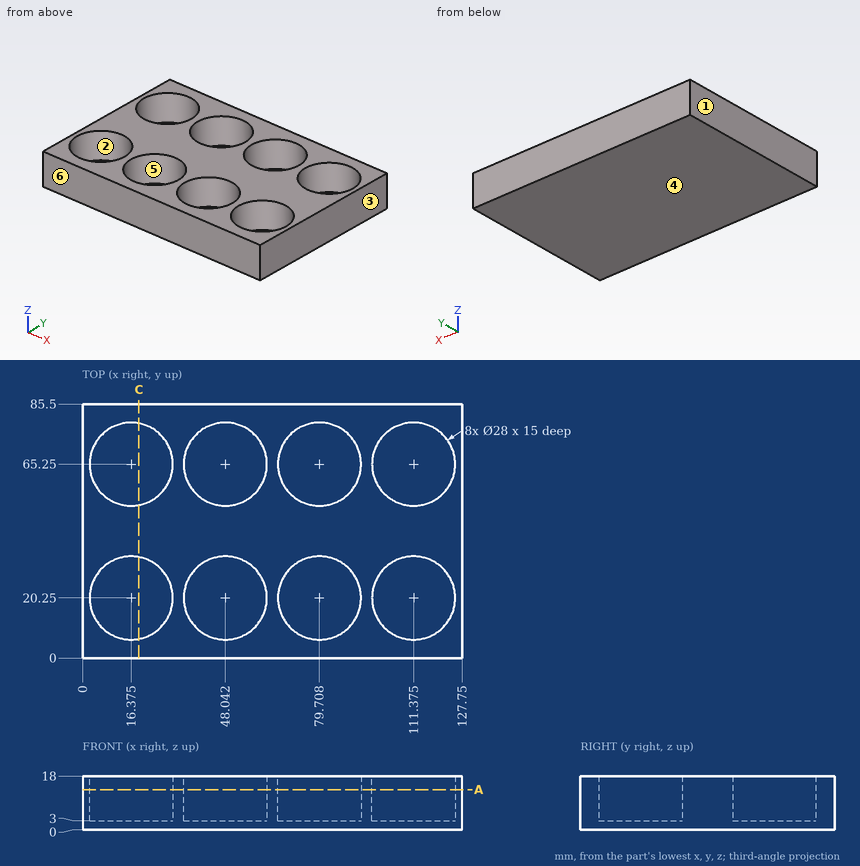
The figure shows three views and two pictorial views of one solid part (mm, origin at its lowest corner). Answer the questions. A direction names the side the tool comes from. Round coordinates to 2 decimals unless told otherwise and drop trailing zeros. Write each loop counter-clockwise with the first axis right and the second up, starting at its lowest first coordinate (ties: lowest second). Pieces come first, ordered by that corner, then holes. Notation, with made-up numbers: (-0.5, 4) - (6.5, 4) arc R27 cw to (6.5, 23) - close; hole circle Ø6 at (72.25, 57.25). An arc over 180 degrees is marked (long way). One line per question, with ' | ' between items. Start each with the question number.
1. Section A-A (z = 13.5) is taken. Give the number of separate pieces and of enclosed holes in the cut face, and give its area (3 significant figures).
2. For a pull along X with two mould halves and no side action, classify the marked faces 1, 2, 3 and 4 as +X half, -X half, draft (parallel to the pull), parting line (faces both ways), or undercut.
3. Find the intervals of material crossed by probe 1 along Y at (x, z) = (48.5, 16); probe 2 along Y at (x, z) = (118, 15.25); probe 3 along Z at (x, y) = (68, 17.5), in increasing order. Write a range as [from, to].
4. For the marked faces 5 and 6, determine the directions among +Z, -Z, +X, -X, +Y, -Y from which every point of the face is accessible in a straight line to the end or side of a thin tool.
5. Section C-C (x = 19) is taken. Determine the outline of the cut face in (y, z), and give its area (3 significant figures).
6. Each of these flat-tipped pins is pushed along its axis until it touches: pin 1 (14 mm diameter, centred on x = 75.5, y = 69, fed in from +Z); pin 2 (17 mm diameter, centred on x = 48.04, y = 20.25, fed in from -Z). Where does it stop, or does it pass through?
Filled in:
1) separate pieces: 1 | enclosed holes: 8 | area: 6,000 mm²
2) face 1: -X half | face 2: undercut | face 3: +X half | face 4: draft
3) probe 1: [0, 6.26], [34.24, 51.26], [79.24, 85.5] | probe 2: [0, 7.92], [32.58, 52.92], [77.58, 85.5] | probe 3: [0, 3]
4) face 5: +Z | face 6: +Z, -Z, +X, -X, -Y
5) outline: (0, 0) - (85.5, 0) - (85.5, 18) - (79, 18) - (79, 3) - (51.5, 3) - (51.5, 18) - (34, 18) - (34, 3) - (6.5, 3) - (6.5, 18) - (0, 18) - close | area: 714 mm²
6) pin 1: z = 3 | pin 2: z = 0
